The listing builds one solid part. Answer for the finished solid, in the listing's coordinates (mm). A direction names the side the tool comes from. Give positions to 0.01 mm unless a question says otherwise; leave off trailing zeros. Write each loop counter-clockwise with the first axis right and the second up, starting at its lowest first coordinate (ties: lowest second). Pieces come first, ordered by that corner, then holes. Notation, with made-up numbers: M 52,-25 L 81,-25 A24 ccw 81,3 Z; hole C -6,-19.75 d11. An arc over 180 degrees is marked long. Return JSON: item names as keys, results as strings.
from build123d import *

# Parameters (mm, degrees)
BOX014_W          = 6
BOX014_H          = 1.5
BOX014_DEPTH      = 12
CYLINDER005_R     = 3
CYLINDER005_DEPTH = 14


with BuildPart() as cube:
    # Box014 → Box014 (new body)
    with BuildSketch(Plane(origin=(-3, -7.44, 8.1), x_dir=(1, 0, 0), z_dir=(0, -1, 0))):
        with Locations((3, 0.75)):
            Rectangle(BOX014_W, BOX014_H)
    extrude(amount=BOX014_DEPTH)


with BuildPart() as shaft:
    # Cylinder005 → Cylinder005 (new body)
    with BuildSketch(Plane(origin=(0, -5.44, 6.6), x_dir=(1, 0, 0), z_dir=(0, -1, 0))):
        Circle(CYLINDER005_R)
    extrude(amount=CYLINDER005_DEPTH)

    # Cut: cut Cube
    add(cube.part, mode=Mode.SUBTRACT)


solid = shaft.part
Item 1: A cutting plane is placed at A-A, the plane x = 0. Write down the section's boundary in (y, z), plus the area to 3 significant figures.
Geometry results:
{"outline": "M -19.44,3.6 L -5.44,3.6 L -5.44,9.6 L -7.44,9.6 L -7.44,8.1 L -19.44,8.1 Z", "area": "66.0 mm2"}
Item 2: A cutting plane is placed at D-D, the plane x = -0.85. Write down the section's boundary in (y, z).
Geometry results:
{"outline": "M -19.44,3.72 L -5.44,3.72 L -5.44,9.48 L -7.44,9.48 L -7.44,8.1 L -19.44,8.1 Z"}
Item 3: Which of the six approach directions +Z, -Z, +X, -X, +Y, -Y give full straight-line access (tool end or side, diameter ignored) to faces 1 (the flat face through (0, -7.44, 9)), 2 (the flat face through (0, -19.44, 6))?
Geometry results:
{"face 1": "+Z, +X, -X, -Y", "face 2": "+Z, -Z, +X, -X, -Y"}
Item 4: Given pin 1 Ø1.6 at (x, z) = (0, 9) entering from -Y; pin 2 Ø1 at (x, y) = (-1.5, -14) entering from +Z, each flat-ended and moving along its own axis, determine where each tip first touches the part or whether it passes through.
Geometry results:
{"pin 1": "stops at y = -7.44", "pin 2": "stops at z = 8.1"}
Item 5: Find the intervals of material crossed by line 1 (Y direction, x = -1.45, z = 8.15); line 2 (X direction, y = -12, z = 5.1); line 3 (Z direction, x = 0.95, y = -10.25), in increasing order.
Geometry results:
{"line 1": "y = -7.44 to -5.44", "line 2": "x = -2.6 to 2.6", "line 3": "z = 3.75 to 8.1"}
Item 6: A cutting plane is placed at B-B, the plane y = -17.25. Write down the section's boundary in (x, z).
Geometry results:
{"outline": "M -2.6,8.1 A3 ccw long 2.6,8.1 Z"}
Item 7: A cutting plane is placed at C-C, the plane z = 7.4. Write down the section's boundary in (x, y).
Geometry results:
{"outline": "M -2.89,-19.44 L 2.89,-19.44 L 2.89,-5.44 L -2.89,-5.44 Z"}
